Input: dimensioned drawing with shaded views. Units: mm. Origin: part minimum x, y, z. A direction names the side the tool comes from. Give positions to 0.01 mm unless a question says otherwise; leave off trailing zeros. Write each loop counter-clockwise with the first axis right and the second up, starting at its lowest first coordinate (ties: lowest second). Pieces come first, ordered by that corner, then holes. Notation, with made-up numbers: (33.25, 12.5) -> (83.25, 12.5) arc R24 cw to (83.25, 22.5) -> close; hole circle Ø1 at (-36.5, 77.5). An arc over 180 degrees is marked (long way). Answer in a Markdown table with one row per item. Add a question column.
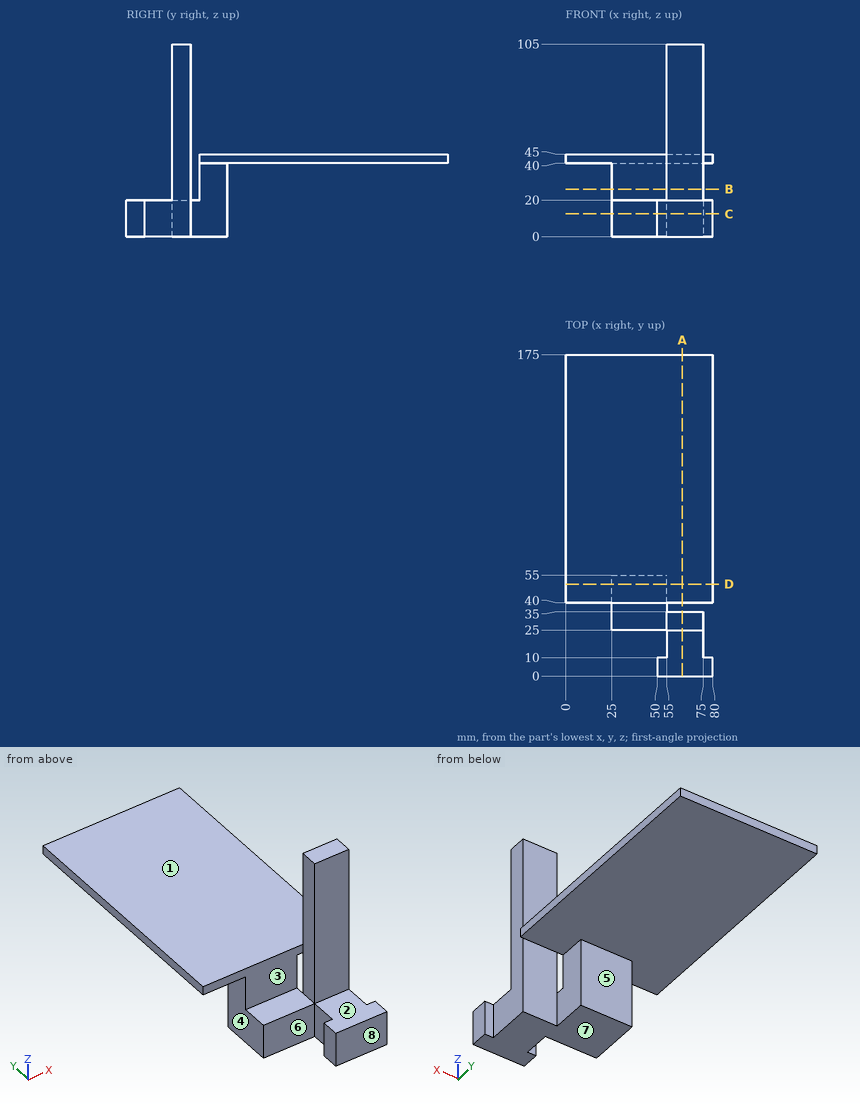
Q1. Line query: probe 1 along Z at (x, y) = (69, 133.5); probe 2 along Y at (x, z) = (64, 73.5); probe 3 along X at (y, z) = (26, 24). Output: solid intervals per line, ascending. Write a range as from..to.
Q2. Section C-C on z = 12.5. Return loops of the section in (x, y).
Q3. Access query for the marked faces 1, 2, 3 and 4. Directions: +Z, -Z, +X, -X, +Y, -Y. A direction counts if a zero-diameter tool reaches every point of the face in a straight line with its end or side. Return the directions, or none.
Q4. Pull-direction query (Y, two-part tool) for the marked faces 5, 6, 7 and 8; classes: +Y half, -Y half, draft (parallel to the pull), parting line (faces both ways), or undercut.
Q5. Section A-A on x = 63.5. Return loops of the section in (y, z).
Q6. Section D-D on y = 50. Return loops of the section in (x, z), and give its area (3 significant figures).
Q7. Section B-B on z = 26. Return loops of the section in (x, y).
Q8. Contact query for flat-ended pins moving along their axis: pin 1 Ø10 at (x, z) = (61, 74.5) entering from +Y; pin 2 Ø5 at (x, z) = (55, 25.5) entering from +Y; pin 3 Ø16 at (x, z) = (36, 14.5) entering from -Y. Output: stop coordinate, or through.
Checks:
| question | item | result |
|---|---|---|
| 1 | probe 1 | 40..45 |
| 1 | probe 2 | 25..35 |
| 1 | probe 3 | 55..75 |
| 2 | outline | (25, 25) -> (55, 25) -> (55, 10) -> (50, 10) -> (50, 0) -> (80, 0) -> (80, 10) -> (75, 10) -> (75, 35) -> (55, 35) -> (55, 55) -> (25, 55) -> close |
| 3 | face 1 | +Z, +X, -X, +Y |
| 3 | face 2 | +Z, +X, -X, -Y |
| 3 | face 3 | +Z, +X, -X |
| 3 | face 4 | -Z, -X, +Y, -Y |
| 4 | face 5 | +Y half |
| 4 | face 6 | undercut |
| 4 | face 7 | draft |
| 4 | face 8 | -Y half |
| 5 | outline | (0, 0) -> (35, 0) -> (35, 105) -> (25, 105) -> (25, 20) -> (0, 20) -> close; (40, 40) -> (175, 40) -> (175, 45) -> (40, 45) -> close |
| 6 | outline | (0, 40) -> (25, 40) -> (25, 0) -> (55, 0) -> (55, 40) -> (80, 40) -> (80, 45) -> (0, 45) -> close |
| 6 | area | 1,600 mm^2 |
| 7 | outline | (25, 40) -> (55, 40) -> (55, 55) -> (25, 55) -> close; (55, 25) -> (75, 25) -> (75, 35) -> (55, 35) -> close |
| 8 | pin 1 | y = 35 |
| 8 | pin 2 | y = 55 |
| 8 | pin 3 | y = 25 |
